Source: CAD feature listing. Evaluate the final solid. Frame: model axes, mm. Face numbers are marked on the shaded views. A direction names the side the tool comes from. Give positions to 0.01 mm unless a question says otherwise; leave off trailing zeros. Loops run counter-clockwise (first coordinate to the right, second up) from the corner with the lowest first, then second, coordinate; pieces in that order, holes last. Notation, with made-up numbers: (62.25, 31.5) -> (106.25, 31.5) arc R28 cw to (106.25, 64.5) -> close; hole circle Ø4 at (-6, 34.25). An arc over 180 degrees is marked (long way). Return JSON: item names as keys, results as strings. Group by question number.
(1) Cut plane A-A on y = 0. Return loops of the section in (x, z), then the cut area to 3 significant figures.
(2) Ray query, line 1 (Y direction, x = 27, z = 31); line 2 (Y direction, x = 27.5, z = 6); line 3 (X direction, y = -1, z = 2.5). Return the intervals inside material, ascending. Write a range as from..to.
(3) Draft query along Y for the marked faces 1, 2 and 3. Return one class per face: released by +Y, released by -Y, zero draft, split by the parting line, or undercut.
(4) Cut plane B-B on x = 27.5. Return loops of the section in (y, z).
(5) Pin query (flat end, axial travel): pin 1 (9 mm diameter, centred on x = 29.5, y = -0.5, fed in from +Z). Return the tip coordinate at first contact, or that it passes through.
(6) Access query for the marked faces 4 and 5. Directions: +Z, -Z, +X, -X, +Y, -Y. A direction counts if a zero-diameter tool reaches every point of the face in a straight line with its end or side. Return the directions, or none.
(7) Cut plane C-C on z = 5. Return loops of the section in (x, y).
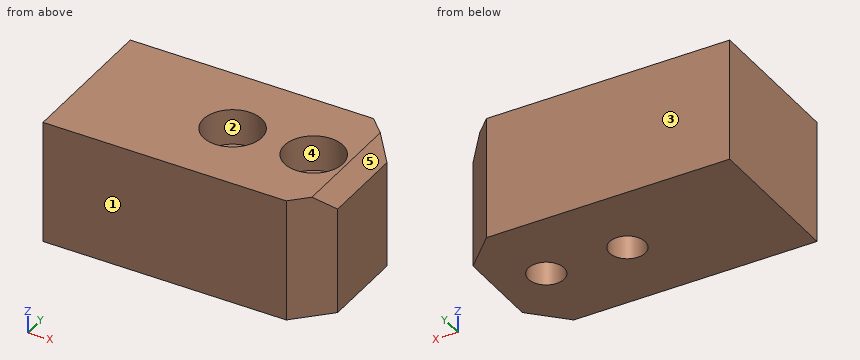
```python
from build123d import *

# Parameters (mm, degrees)
SKETCH_1_W                = 85
SKETCH_1_H                = 46
EXTRUDE_1_DEPTH           = 38
HOLE_WIZARD_1_D           = 11
HOLE_WIZARD_1_CBORE_D     = 18
HOLE_WIZARD_1_CBORE_DEPTH = 11
CHAMFER_1_SIZE            = 10
CHAMFER_2_SIZE            = 5


with BuildPart() as part:
    # 草图1 → 凸台-拉伸1 (new body)
    with BuildSketch(Plane.XY):
        Rectangle(SKETCH_1_W, SKETCH_1_H)
    extrude(amount=EXTRUDE_1_DEPTH)

    # 打孔尺寸(%根据)内六角圆柱头螺钉的类型1 (through all)
    with Locations(Plane.XY.offset(38)):
        with Locations((2.5, 0), (27.5, 0)):
            CounterBoreHole(HOLE_WIZARD_1_D / 2, HOLE_WIZARD_1_CBORE_D / 2, HOLE_WIZARD_1_CBORE_DEPTH)

    # 倒角1
    chamfer_1_edges = [part.edges().sort_by_distance(p)[0] for p in [
        (42.5, 23, 19),
        (42.5, -23, 19),
    ]]
    chamfer(chamfer_1_edges, length=CHAMFER_1_SIZE)

    # 倒角2
    chamfer_2_edges = [part.edges().sort_by_distance(p)[0] for p in [
        (42.5, 0, 38),
    ]]
    chamfer(chamfer_2_edges, length=CHAMFER_2_SIZE)


solid = part.part
```
Answers:
{
 "1": {"outline": "(-42.5, 0) -> (-3, 0) -> (-3, 27) -> (-6.5, 27) -> (-6.5, 38) -> (-42.5, 38) -> close; (8, 0) -> (22, 0) -> (22, 27) -> (18.5, 27) -> (18.5, 38) -> (11.5, 38) -> (11.5, 27) -> (8, 27) -> close; (33, 0) -> (42.5, 0) -> (42.5, 33) -> (37.5, 38) -> (36.5, 38) -> (36.5, 27) -> (33, 27) -> close", "area": "2,230 mm²"},
 "2": {"line 1": "-23..-8.99, 8.99..23", "line 2": "-23..-5.5, 5.5..23", "line 3": "-42.5..-2.91, 7.91..22.09, 32.91..42.5"},
 "3": {"face 1": "released by -Y", "face 2": "undercut", "face 3": "released by +Y"},
 "4": {"outline": "(-23, 0) -> (-5.5, 0) -> (-5.5, 27) -> (-9, 27) -> (-9, 38) -> (-23, 38) -> close; (5.5, 0) -> (23, 0) -> (23, 38) -> (9, 38) -> (9, 27) -> (5.5, 27) -> close"},
 "5": {"pin 1": "z = 27"},
 "6": {"face 4": "+Z", "face 5": "+Z, +X, +Y, -Y"},
 "7": {"outline": "(-42.5, -23) -> (32.5, -23) -> (42.5, -13) -> (42.5, 13) -> (32.5, 23) -> (-42.5, 23) -> close; hole circle Ø11 at (2.5, 0); hole circle Ø11 at (27.5, 0)"}
}
